The model under review builds one solid part; all positions refer to its coordinate system, in mm. A direction names the side the tool comes from. Round coordinates to 2 decimals unless told otherwise and drop trailing zeros. Order: outer loops, then holes, each group sorted by start corner. A loop starts at its lowest first (then second) coordinate and runs counter-clockwise, first axis right, second up.
1) Clearance check with flat-ended pins moving along their axes: P1, Ø6.5, axis at x = 8.5, y = 7, coming from the -Z side; P2, Ø3, axis at y = -3.5, z = -4.5, coming from the +X side; P3, Ø4, axis at x = 7.5, z = -3.5, coming from the -Y side; P4, Ø0.5, axis at x = -9.5, y = 0, coming from the -Z side. State where each tip first meets the part, or that it passes through.
2) Machinability: for faces 4 (the face through (8.314, 3.35, 2.623)), 5 (the face through (-5, 0, -3)), 6 (the face through (4.699, 9.715, -2.535)), which of the approach directions +Z, -Z, +X, -X, +Y, -Y give a long, thin tool a straight path to every point of the face, cutting with its end or side? Answer none if there is none.
3) Consider section C-C (x = -2.75). Give the boundary of the cut face in (y, z), then the cut area to 3 significant figures.
4) Consider section D-D (z = -1). Give the boundary of the cut face in (x, y).
5) Consider section B-B (z = 5.25). Give the boundary of the cut face in (x, y), then the cut area to 3 significant figures.
6) To check wall thickness, follow L1, parallel to Y at x = -8, z = 4.4; L2, parallel to X at y = -7.5, z = 4.05; L3, parallel to Y at x = 8, z = 2.6. State the ranges of each line that lie inside material, in increasing order.
7) Mouldability with a two-part tool opening along Y and no side actions: class faces 1 (the face through (-8.314, 3.419, 2.569)), 2 (the face through (-10, -7, 0)), 3 (the face through (-11.5, 9.43, 2.84)) as pulls with the +Y half, pulls with the -Y half, needs draft (parallel to the pull), parting line crosses it, or undercut.
8) Consider section A-A (x = -8). Give the boundary of the cut face in (y, z), then the cut area to 3 significant figures.
Autodesk Fusion 360 part; units mm, degrees
sketch "Sketch1" plane through (0, 0, 0) normal (0, 0, 1) x (1, 0, 0) in component "x_carriage_pivot_block"
  line L0 (12.1, 10) -> (-12.1, 10)
  line L1 (-12.1, 10) -> (-12.1, -10)
  line L2 (-12.1, -10) -> (12.1, -10)
  line L3 (12.1, -10) -> (12.1, 10)
  line L4 (12.1, 10) -> (-12.1, -10) construction
  line L5 (-12.1, 10) -> (12.1, -10) construction
  dimension "d1" = 24.2
  dimension "d2" = 20
extrude "Extrude1" add sketch "Sketch1" along normal blind 6 in component "x_carriage_pivot_block"
sketch "Sketch2" plane through (0, 0, 0) normal (0, 0, -1) x (1, 0, 0) in component "x_carriage_pivot_block"
  line L0 (12.1, -10) -> (12.1, 10)
  line L1 (12.1, 10) -> (-12.1, 10)
  line L2 (-12.1, 10) -> (-12.1, -10)
  line L3 (-12.1, -10) -> (12.1, -10)
  line L4 (5, 10) -> (-5, 10)
  line L5 (-5, 10) -> (-5, -10)
  line L6 (-5, -10) -> (5, -10)
  line L7 (5, -10) -> (5, 10)
  line L8 (5, 10) -> (-5, -10) construction
  line L9 (-5, 10) -> (5, -10) construction
  dimension "d5" = 10
  dimension "d6" = 20
extrude "Extrude2" add sketch "Sketch2" along normal blind 8 contours L1 L3 L4 L5 L6 L7 in component "x_carriage_pivot_block"
sketch "Sketch3" plane through (0, 0, 0) normal (1, 0, 0) x (0, 1, 0) in component "x_carriage_pivot_block"
  line L0 (10, 0) -> (10, 6) construction
  line L1 (10, 6) -> (-10, 6) construction
  line L2 (-10, 6) -> (-10, 0) construction
  line L3 (-10, 0) -> (-10, -8) construction
  line L4 (-10, -8) -> (10, -8) construction
  line L5 (10, -8) -> (10, 0) construction
  line L6 (-0.5, -2.8) -> (0.5, -2.8)
  arc A0 (0.5, -2.8) -> (0.5, 0.8) centre (0.5, -1) ccw
  line L7 (0.5, 0.8) -> (-0.5, 0.8)
  arc A1 (-0.5, 0.8) -> (-0.5, -2.8) centre (-0.5, -1) ccw
  line L8 (-0.5, -1) -> (0.5, -1) construction
  line L9 (0, 6) -> (0, -8) construction
  line L10 (-0.5, -5.61) -> (0.5, -5.61)
  arc A2 (0.5, -5.61) -> (0.5, 3.61) centre (0.5, -1) ccw
  line L11 (0.5, 3.61) -> (-0.5, 3.61)
  arc A3 (-0.5, 3.61) -> (-0.5, -5.61) centre (-0.5, -1) ccw
  line L12 (-0.5, -1) -> (0.5, -1) construction
  point P0 (0, -1)
  dimension "d9" = 3.6
  dimension "d11" = 1
  dimension "d12" = 9.22
extrude "Extrude3" cut sketch "Sketch3" along normal through all and the other way through all contours L6 A0 L7 A1 in component "x_carriage_pivot_block"
extrude "Extrude4" cut sketch "Sketch3" along normal through all from surface at 5 in component "x_carriage_pivot_block"
extrude "Extrude5" cut sketch "Sketch3" against normal through all from surface at -5 in component "x_carriage_pivot_block"
sketch "Sketch4" plane through (0, 0, 6) normal (0, 0, 1) x (-1, 0, 0) in component "x_carriage_pivot_block"
  line L0 (-12.1, 10) -> (-12.1, -10)
  line L1 (-12.1, -10) -> (12.1, -10)
  line L2 (12.1, -10) -> (12.1, 10)
  line L3 (12.1, 10) -> (-12.1, 10)
  circle A0 centre (8, -7.5) radius 1.7
  line L4 (0, 0) -> (0, -13) construction
  line L5 (0, 0) -> (-15, 0) construction
  circle A1 centre (-8, -7.5) radius 1.7
  circle A2 centre (8, 7.5) radius 1.7
  circle A3 centre (-8, 7.5) radius 1.7
  dimension "d19" = 3.4
  dimension "d20" = 16
  dimension "d21" = 15
extrude "Extrude6" cut sketch "Sketch4" against normal through all contours A0 | A1 | A2 | A3 in component "x_carriage_pivot_block"
fillet "Fillet1" radius 3 2 edges at (0, -10, -8) (0, 10, -8) in component "x_carriage_pivot_block"
fillet "Fillet2" radius 1 10 edges at (-5, 10, -2.5) (-5, 9.1213, -7.1213) (-5, 0, -8) (-5, -9.1213, -7.1213) (-5, -10, -2.5) (5, 10, -2.5) (5, 9.1213, -7.1213) (5, 0, -8) (5, -9.1213, -7.1213) (5, -10, -2.5) in component "x_carriage_pivot_block"
fillet "Fillet3" radius 1.2 6 edges at (-12.1, 3.3846, 2.596) (-12.1, 0, 3.61) (-12.1, -3.3846, 2.596) (12.1, -3.3846, 2.596) (12.1, 0, 3.61) (12.1, 3.3846, 2.596) in component "x_carriage_pivot_block"
fillet "Fillet4" radius 0.8 6 edges at (-5, 3.3846, 2.596) (-5, 0, 3.61) (-5, -3.3846, 2.596) (5, -3.3846, 2.596) (5, 0, 3.61) (5, 3.3846, 2.596) in component "x_carriage_pivot_block"
fillet "Fillet5" radius 2 4 edges at (-12.1, 10, 3) (-12.1, -10, 3) (12.1, -10, 3) (12.1, 10, 3) in component "x_carriage_pivot_block"
chamfer "Chamfer1" distance 0.4 angle 45 8 edges at (12.1, 0, 6) (11.5142, 9.4142, 6) (0, 10, 6) (-11.5142, 9.4142, 6) (-12.1, 0, 6) (-11.5142, -9.4142, 6) (0, -10, 6) (11.5142, -9.4142, 6) in component "x_carriage_pivot_block"
component "x_carriage_pivot_block" placed x (1, 0, 0) y (0, 1, 0) z (0, 0, 1) at (0, 0, 0)
equation "pivot_movement = 1 mm"
equation "d11 = pivot_movement"
equation "d12 = ( 4.61 * 2 ) * 1 mm"
equation "d19 = ( 1.7 * 2 ) * 1 mm"
equation "d33 = chamfer"
equation "chamfer = 0.4 mm"
Answer below:
1. P1: stops at z = 0
1. P2: stops at x = 5
1. P3: passes through
1. P4: stops at z = 3.61
2. face 4: -Z, +X
2. face 5: -Z, -X
2. face 6: -Z, +X, +Y
3. outline: (-10, -5) arc R3 ccw to (-7, -8) - (7, -8) arc R3 ccw to (10, -5) - (10, 5.6) - (9.6, 6) - (-9.6, 6) - (-10, 5.6) - close; hole (-0.5, -2.8) - (0.5, -2.8) arc R1.8 ccw to (0.5, 0.8) - (-0.5, 0.8) arc R1.8 ccw to start
3. area: 262 mm2
4. outline: (-5, -9) arc R1 ccw to (-4, -10) - (4, -10) arc R1 ccw to (5, -9) - (5, -2.3) - (-5, -2.3) - close; (-5, 2.3) - (5, 2.3) - (5, 9) arc R1 ccw to (4, 10) - (-4, 10) arc R1 ccw to (-5, 9) - close
5. outline: (-12.1, -8) arc R2 ccw to (-10.1, -10) - (10.1, -10) arc R2 ccw to (12.1, -8) - (12.1, 8) arc R2 ccw to (10.1, 10) - (-10.1, 10) arc R2 ccw to (-12.1, 8) - close; hole circle Ø3.4 at (-8, -7.5); hole circle Ø3.4 at (-8, 7.5); hole circle Ø3.4 at (8, -7.5); hole circle Ø3.4 at (8, 7.5)
5. area: 444 mm2
6. L1: y = -10 to -9.2, -5.8 to 5.8, 9.2 to 10
6. L2: x = -12.1 to -9.7, -6.3 to 6.3, 9.7 to 12.1
6. L3: y = -10 to -9.2, -5.8 to -3.38, 3.38 to 5.8, 9.2 to 10
7. face 1: undercut
7. face 2: needs draft
7. face 3: pulls with the +Y half
8. outline: (-10, 0) - (-9.2, 0) - (-9.2, 6) - (-9.6, 6) - (-10, 5.6) - close; (-5.8, 0) - (-5, 0) arc R4.61 cw to (-0.5, 3.61) - (0.5, 3.61) arc R4.61 cw to (5, 0) - (5.8, 0) - (5.8, 6) - (-5.8, 6) - close; (9.2, 0) - (10, 0) - (10, 5.6) - (9.6, 6) - (9.2, 6) - close
8. area: 51.2 mm2
